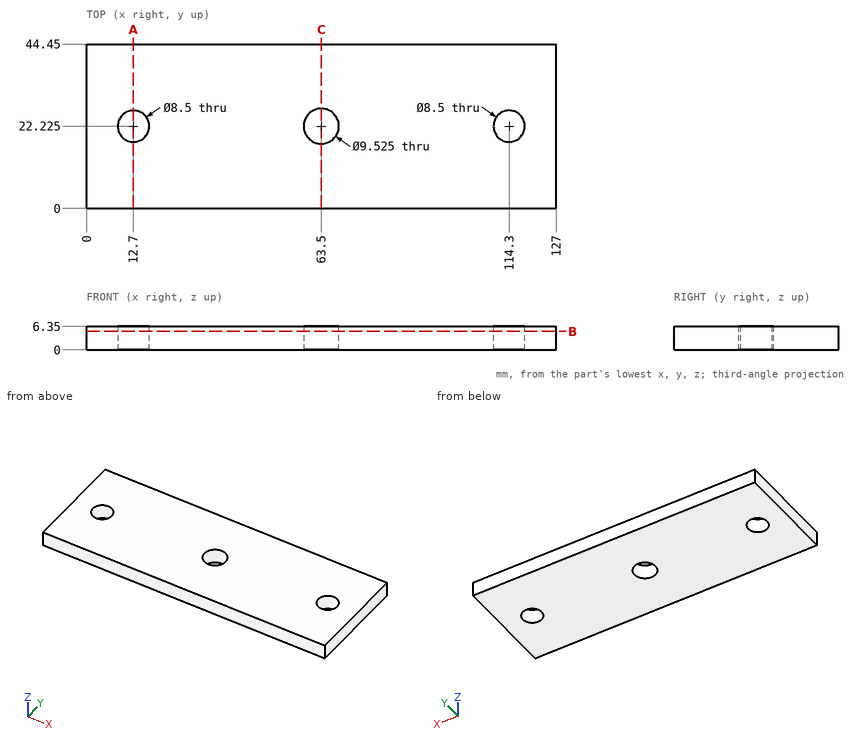
Could you check a few things on this drawing? It's one solid part, dimensions in mm from its lowest x, y, z. Give positions to 0.01 mm unless a question says otherwise; leave off trailing zeros. Write each loop counter-clockwise with the first axis right and the second up, starting at its lowest first coordinate (ties: lowest second). Pieces come first, ordered by that corner, then holes. Notation, with made-up numbers: M 30.5,-26.75 L 51.5,-26.75 A23 ccw 51.5,6.25 Z; hole C -29.75,7.25 d8. An arc over 180 degrees is marked long. Put each result on its own line as item: value. Start each with the question number.
Item 1: If we section it at B-B, the plane z = 5: Count the separate pieces of the cut face and the enclosed holes in it, then the cut area to 3 significant figures.
Item 2: If we section it at A-A, the plane x = 12.7: Write out the boundary of the cut face in (y, z) (3 decimals), then the cut area to 3 significant figures.
Item 3: If we section it at C-C, the plane x = 63.5: Write out the boundary of the cut face in (y, z).
Item 4: I need wall thicknesses on L1, parallel to Y at x = 114.3, z = 4.25 (3 decimals); L2, parallel to X at y = 23.5, z = 2.75; L3, parallel to Y at x = 63.5, z = 2.25. Which ranges of each line are inside material? Lowest first, please. Write a range as from..to.
Item 5: Will this pin go through, and if not, where does the flat tip stop? pin 1 (7.5 mm diameter, centred on x = 114.3, y = 22.225, fed in from -Z).
Values:
1. separate pieces: 1
1. enclosed holes: 3
1. area: 5,460 mm²
2. outline: M 0,0 L 17.975,0 L 17.975,6.35 L 0,6.35 Z; M 26.475,0 L 44.45,0 L 44.45,6.35 L 26.475,6.35 Z
2. area: 228 mm²
3. outline: M 0,0 L 17.46,0 L 17.46,6.35 L 0,6.35 Z; M 26.99,0 L 44.45,0 L 44.45,6.35 L 26.99,6.35 Z
4. L1: 0..17.975, 26.475..44.45
4. L2: 0..8.65, 16.75..58.91, 68.09..110.25, 118.35..127
4. L3: 0..17.46, 26.99..44.45
5. pin 1: through
